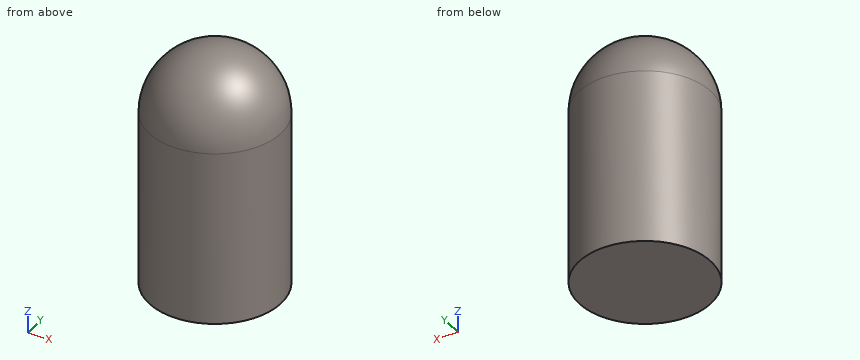
```python
from build123d import *

# Parameters (mm, degrees)
F0_R     = 155
F1_DEPTH = 405
F4_R     = 148
F5_DEPTH = 405
F6_R     = 155
F6_R_2   = 148
F7_DEPTH = 5


with BuildPart() as f1:
    # F0 (on Top) → F1 (new body)
    with BuildSketch(Plane.XY):
        Circle(F0_R)
    extrude(amount=F1_DEPTH)

    # F2 (on face) → F3 (revolve)
    with BuildSketch(Plane.XY.offset(405)):
        with BuildLine():
            Line((0, 148), (0, 155))
            ThreePointArc((0, 155), (-155, 0), (0, -155))
            Line((0, -155), (0, -148))
            ThreePointArc((0, -148), (-148, 0), (0, 148))
        make_face()
    revolve(axis=Axis((0, -77.5, 405), (0, -1, 0)))

    # F4 (on face) → F5 (cut)
    with BuildSketch(Plane(origin=(0, 0, 0), x_dir=(1, 0, 0), z_dir=(0, 0, -1))):
        Circle(F4_R)
    extrude(amount=-F5_DEPTH, mode=Mode.SUBTRACT)

    # F6 (on face) → F7 (join)
    with BuildSketch(Plane(origin=(0, 0, 0), x_dir=(1, 0, 0), z_dir=(0, 0, -1))):
        Circle(F6_R)
        Circle(F6_R_2)
    extrude(amount=F7_DEPTH)


solid = f1.part
```
Design review of the part built by this model. Coordinates are the model's own, in mm. Round coordinates to 2 decimals unless told otherwise and drop trailing zeros. Write each loop counter-clockwise with the first axis right and the second up, starting at its lowest first coordinate (ties: lowest second). Pieces come first, ordered by that corner, then holes. Notation, with made-up numbers: (-31, -7) -> (-24, -7) arc R28 cw to (-24, 19) -> close; hole circle Ø5 at (89.5, 42.25). An arc over 180 degrees is marked (long way). Write item = value, one per line. Start each with the question number.
1) Take a section at A-A, the plane x = 0. State the section outline as (y, z) points.
2) Wall thickness on probe 1 along Y at (x, z) = (0, 205); probe 2 along Z at (x, y) = (-14, -69): over which ranges is each line inside the solid? List them lowest first. Write a range as from..to.
3) Clearance check with flat-ended pins moving along their axes: pin 1 (2 mm diameter, centred on x = 1, z = 337, fed in from -Y); pin 2 (10 mm diameter, centred on x = 70.5, z = 300, fed in from -Y); pin 3 (2 mm diameter, centred on y = -37, z = 498, fed in from +X). State where each tip first meets the part, or that it passes through.
4) Take a section at C-C, the plane z = 163.5. State the section outline as (x, y) points, plus the area to 3 significant figures.
Results list:
q1.outline = (-155, -5) -> (155, -5) -> (155, 405) arc R155 ccw to (-155, 405) -> close; hole (-148, 0) -> (148, 0) -> (148, 405) arc R148 ccw to (-148, 405) -> close
q2.probe_1 = -155..-148, 148..155
q2.probe_2 = -5..0, 535.18..543.09
q3.pin_1 = -155
q3.pin_2 = -140.48
q3.pin_3 = 119.19
q4.outline = circle Ø310 at (0, 0); hole circle Ø296 at (0, 0)
q4.area = 6,660 mm²
